Read the model definition and answer for the solid it produces. Units are mm, in the model's axes. A direction names the side the tool comes from. Give positions to 0.01 mm unless a question says otherwise; leave off trailing zeros. Loops run counter-clockwise (first coordinate to the right, second up) from the corner with the lowest first, then second, coordinate; pieces in that order, holes last. Notation, with made-up numbers: (22.25, -37) -> (50.25, -37) arc R22 cw to (50.25, -2) -> close; hole circle Ø2 at (-18, -13). An arc over 180 degrees is marked (long way). Write each question's results on one line, items separated by ' | '. Start each with the question number.
Item 1: Determine the mould class of faces 4 (the cylindrical face through (7.647, 0.024, -3.451)), 5 (the flat face through (0, -4, -7)) for opening direction X: +X half, -X half, draft (parallel to the pull), parting line (faces both ways), or undercut.
Item 2: Each of these flat-tipped pins is pushed along its axis until it touches: P1, Ø12, axis at x = -3, z = 7.5, coming from the -Y side; P2, Ø1, axis at y = 4, z = 0, coming from the -X side; P3, Ø1.5, axis at y = 7.5, z = 7.5, coming from the +X side; P4, Ø1, axis at x = -5, z = 10, coming from the +Y side. Where does it stop, or does it pass through?
Item 3: Find the intervals of material crossed by line 1 (Y direction, x = 0, z = -1.75); line 2 (Z direction, x = -7, y = -0.25); line 3 (X direction, y = -1.25, z = 2.75), in increasing order.
Item 4: Which of the six approach directions +Z, -Z, +X, -X, +Y, -Y give full straight-line access (tool end or side, diameter ignored) to faces 1 (the flat face through (2, -2, 0)), 2 (the flat face through (-0.1, 2.4, 15)), 3 (the cylindrical face through (-5.453, -1.952, 7.934))?
Item 5: Section B-B on x = -7.1 is taken. Write down the section's boundary in (y, z), and give its area (3 significant figures).
Item 6: Section A-A on z = -5 is taken. Write down the section's boundary in (x, y), and give its area (3 significant figures).
Item 7: Section C-C on x = 7.1 is taken. Write down the section's boundary in (y, z), and give its area (3 significant figures).
```python
from build123d import *

# Parameters (mm, degrees)
ESBO_O1_R                = 10
ESBO_O1_R_2              = 2.25
RESSALTO_EXTRUS_O1_DEPTH = 15
ESBO_O2_R                = 2
CORTE_EXTRUS_O1_DEPTH    = 10
ESBO_O3_R                = 10
ESBO_O3_R_2              = 0.547725274
ESBO_O3_R_3              = 3.7
RESSALTO_EXTRUS_O2_DEPTH = 7


with BuildPart() as part:
    # Esboço1 → Ressalto-extrusão1 (new body)
    with BuildSketch(Plane.XY):
        Circle(ESBO_O1_R)
        Circle(ESBO_O1_R_2, mode=Mode.SUBTRACT)
    extrude(amount=RESSALTO_EXTRUS_O1_DEPTH)

    # Esboço2 → Corte-extrusão1 (cut)
    with BuildSketch(Plane(origin=(0, 0, 0), x_dir=(0, 0, -1), z_dir=(1, 0, 0))):
        with Locations((-7.5, 0)):
            Circle(ESBO_O2_R)
    extrude(amount=-CORTE_EXTRUS_O1_DEPTH, mode=Mode.SUBTRACT)

    # Esboço3 → Ressalto-extrusão2 (add)
    with BuildSketch(Plane(origin=(0, 0, 0), x_dir=(-1, 0, 0), z_dir=(0, 0, -1))):
        Circle(ESBO_O3_R)
        with Locations((0, 7.1)):
            Circle(ESBO_O3_R_2, mode=Mode.SUBTRACT)
        with Locations((7.1, 0)):
            Circle(ESBO_O3_R_2, mode=Mode.SUBTRACT)
        with Locations((0, -7.1)):
            Circle(ESBO_O3_R_2, mode=Mode.SUBTRACT)
        with Locations((-7.1, 0)):
            Circle(ESBO_O3_R_2, mode=Mode.SUBTRACT)
        Circle(ESBO_O3_R_3, mode=Mode.SUBTRACT)
    extrude(amount=RESSALTO_EXTRUS_O2_DEPTH)


solid = part.part
```
Findings:
1) face 4: undercut | face 5: draft
2) P1: y = -10 | P2: x = -9.37 | P3: x = 7.38 | P4: y = 8.93
3) line 1: -10 to -7.65, -6.55 to -3.7, 3.7 to 6.55, 7.65 to 10 | line 2: 0 to 5.52, 9.48 to 15 | line 3: -9.92 to -1.87, 1.87 to 9.92
4) face 1: -Z | face 2: +Z, +X, -X, +Y, -Y | face 3: -X
5) outline: (-7.04, -7) -> (-0.55, -7) -> (-0.55, 0) -> (0.55, 0) -> (0.55, -7) -> (7.04, -7) -> (7.04, 15) -> (-7.04, 15) -> close; hole circle Ø4 at (0, 7.5) | area: 290 mm2
6) outline: circle Ø20 at (0, 0); hole circle Ø1.1 at (-7.1, 0); hole circle Ø7.4 at (0, 0); hole circle Ø1.1 at (0, -7.1); hole circle Ø1.1 at (0, 7.1); hole circle Ø1.1 at (7.1, 0) | area: 267 mm2
7) outline: (-7.04, -7) -> (-0.55, -7) -> (-0.55, 0) -> (0.55, 0) -> (0.55, -7) -> (7.04, -7) -> (7.04, 15) -> (-7.04, 15) -> close | area: 302 mm2
